CAD build for the part. Positions are in the model's coordinates, mm. A direction names the side the tool comes from. Round coordinates to 2 decimals unless told otherwise and drop trailing zeros. Loops run counter-clockwise (first coordinate to the right, second up) from the corner with the lowest first, then second, coordinate; pieces in that order, holes last.
from build123d import *

# Parameters (mm, degrees)
SKETCH1_R           = 10
SKETCH1_R_2         = 8.7
BOSS_EXTRUDE1_DEPTH = 87
SKETCH2_R           = 10.87
BOSS_EXTRUDE2_DEPTH = 17
SKETCH3_R           = 3.52
BOSS_EXTRUDE3_DEPTH = 7
SKETCH4_R           = 8.7
CUT_EXTRUDE1_DEPTH  = 14
BOSS_EXTRUDE4_START = -0.085517
SKETCH5_R           = 1.305
BOSS_EXTRUDE4_DEPTH = 1.585517
FILLET1_R           = 0.4


with BuildPart() as part:
    # Sketch1 → Boss-Extrude1 (new body)
    with BuildSketch(Plane(origin=(0, 0, 0), x_dir=(1, 0, 0), z_dir=(0, 1, 0))):
        Circle(SKETCH1_R)
        Circle(SKETCH1_R_2, mode=Mode.SUBTRACT)
    extrude(amount=BOSS_EXTRUDE1_DEPTH)

    # Sketch2 → Boss-Extrude2 (add)
    with BuildSketch(Plane.XZ):
        Circle(SKETCH2_R)
    extrude(amount=-BOSS_EXTRUDE2_DEPTH)

    # Sketch3 → Boss-Extrude3 (add)
    with BuildSketch(Plane.XZ):
        Circle(SKETCH3_R)
    extrude(amount=BOSS_EXTRUDE3_DEPTH)

    # Sketch4 → Cut-Extrude1 (cut)
    with BuildSketch(Plane(origin=(0, 17, 0), x_dir=(1, 0, 0), z_dir=(0, 1, 0))):
        Circle(SKETCH4_R)
    extrude(amount=-CUT_EXTRUDE1_DEPTH, mode=Mode.SUBTRACT)

    # Sketch5 → Boss-Extrude4 (add)
    with BuildSketch(Plane(origin=(10, 0, 0), x_dir=(0, 0, -1), z_dir=(1, 0, 0)).offset(BOSS_EXTRUDE4_START)):
        with Locations((0, 51.5)):
            Circle(SKETCH5_R)
    extrude(amount=BOSS_EXTRUDE4_DEPTH)

    # Fillet1
    fillet1_edges = [part.edges().sort_by_distance(p)[0] for p in [
        (-10, 17, 0),
        (-10.87, 17, 0),
        (-10.87, 0, 0),
        (-3.52, 0, 0),
        (-3.52, -7, 0),
    ]]
    fillet(fillet1_edges, radius=FILLET1_R)


solid = part.part
Item 1: Flat gauge pins, fed straight in: P1, Ø3, axis at y = 66, z = 7.5, coming from the +X side; P2, Ø5, axis at y = 2.5, z = 6.5, coming from the +X side; P3, Ø6, axis at y = 63, z = 1, coming from the -X side. Where does each tip first touch, or does it go through?
Verdict:
P1: stops at x = 8
P2: stops at x = 10.11
P3: stops at x = -10
Item 2: Wall check: L1, parallel to X at y = 68.5, z = 0; L2, parallel to Y at x = -2.25, z = 1. Give the ranges that are in metal, low to high.
Verdict:
L1: x = -10 to -8.7, 8.7 to 10
L2: y = -7 to 3
Item 3: Cut at C-C (x = 0). List the corners of the cut face in (y, z).
Verdict:
outline: (-7, -3.12) arc R0.4 ccw to (-6.6, -3.52) - (-0.4, -3.52) arc R0.4 cw to (0, -3.92) - (0, -10.47) arc R0.4 ccw to (0.4, -10.87) - (16.6, -10.87) arc R0.4 ccw to (17, -10.47) - (17, -10.4) arc R0.4 cw to (17.4, -10) - (87, -10) - (87, -8.7) - (3, -8.7) - (3, 8.7) - (87, 8.7) - (87, 10) - (17.4, 10) arc R0.4 cw to (17, 10.4) - (17, 10.47) arc R0.4 ccw to (16.6, 10.87) - (0.4, 10.87) arc R0.4 ccw to (0, 10.47) - (0, 3.92) arc R0.4 cw to (-0.4, 3.52) - (-6.6, 3.52) arc R0.4 ccw to (-7, 3.12) - close
Item 4: Cut at A-A (y = 51.5). List the corners of the cut face in (x, z) (3 decimals), plus the area to 3 significant figures.
Verdict:
outline: (9.914, -1.305) - (11.5, -1.305) - (11.5, 1.305) - (9.914, 1.305) arc R10 ccw (long way) to start; hole circle Ø17.4 at (0, 0)
area: 80.4 mm2
Item 5: 3-axis set-ups, long thin cutter, end or side, ignore diameter. For faces 4 (the flat face through (11.5, 52, 0)), 5 (the flat face through (0, 3, 0)), 6 (the cylindrical face through (10.696, 51, -1.205)), 7 (the cylindrical face through (-0.763, -3.457, -3.436)), 8 (the flat face through (0, -7, 0)): which of +Z, -Z, +X, -X, +Y, -Y reach the whole face in a straight line?
Verdict:
face 4: +Z, -Z, +X, +Y, -Y
face 5: +Y
face 6: +X
face 7: -Y
face 8: +Z, -Z, +X, -X, -Y
Item 6: Mould opens along Z. For faces 1 (the flat face through (-1, 87, 9)), 2 (the cylindrical face through (-1.886, 44.412, 8.493)), 3 (the cylindrical face through (-2.17, 51.71, 9.76)) say: released by +Z, released by -Z, zero draft, split by the parting line, or undercut.
Verdict:
face 1: zero draft
face 2: undercut
face 3: split by the parting line
Item 7: Cut at D-D (y = 14.5). List the corners of the cut face in (x, z).
Verdict:
outline: circle Ø21.74 at (0, 0); hole circle Ø17.4 at (0, 0)
